Geometry check sheet. Reference: the model listing, model coordinates, mm. Face numbers are marked on the shaded views. Coordinates: 2 decimals unless noted, no trailing zeros. Write each loop counter-clockwise with the first axis right and the second up, starting at its lowest first coordinate (ties: lowest second). Pieces come first, ordered by that corner, then holes. Notation, with made-up numbers: (37.25, 70.5) - (64.25, 70.5) arc R21 ccw to (64.25, 94.5) - close; hole circle Ø9 at (-32, 71.5). An arc over 180 degrees is marked (long way). Answer as a JSON object with one key per item and string values. Group by question number.
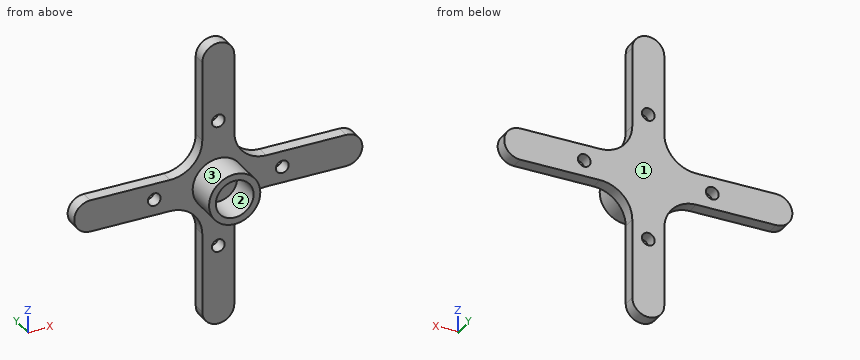
from build123d import *

# Parameters (mm, degrees)
SKETCH1_R           = 1
BOSS_EXTRUDE1_DEPTH = 2
SKETCH2_R           = 4
SKETCH2_R_2         = 2.95
BOSS_EXTRUDE2_DEPTH = 5


with BuildPart() as part:
    # Sketch1 → Boss-Extrude1 (new body)
    with BuildSketch(Plane(origin=(0, 0, 0), x_dir=(1, 0, 0), z_dir=(0, 1, 0))):
        with BuildLine():
            Line((2.5, 20), (2.5, 7.5))
            ThreePointArc((2.5, 7.5), (3.964466094, 3.964466094), (7.5, 2.5))
            Line((7.5, 2.5), (20, 2.5))
            ThreePointArc((20, 2.5), (22.5, 0), (20, -2.5))
            Line((20, -2.5), (7.5, -2.5))
            ThreePointArc((7.5, -2.5), (3.964466094, -3.964466094), (2.5, -7.5))
            Line((2.5, -7.5), (2.5, -20))
            ThreePointArc((2.5, -20), (0, -22.5), (-2.5, -20))
            Line((-2.5, -20), (-2.5, -7.5))
            ThreePointArc((-2.5, -7.5), (-3.964466094, -3.964466094), (-7.5, -2.5))
            Line((-7.5, -2.5), (-20, -2.5))
            ThreePointArc((-20, -2.5), (-22.5, 0), (-20, 2.5))
            Line((-20, 2.5), (-7.5, 2.5))
            ThreePointArc((-7.5, 2.5), (-3.964466094, 3.964466094), (-2.5, 7.5))
            Line((-2.5, 7.5), (-2.5, 20))
            ThreePointArc((-2.5, 20), (0, 22.5), (2.5, 20))
        make_face()
        with Locations(Location((10, 0, 0), (0, 0, 270))):
            Circle(SKETCH1_R, mode=Mode.SUBTRACT)
        with Locations(Location((-10, 0, 0), (0, 0, 270))):
            Circle(SKETCH1_R, mode=Mode.SUBTRACT)
        with Locations(Location((0, 10, 0), (0, 0, 270))):
            Circle(SKETCH1_R, mode=Mode.SUBTRACT)
        with Locations(Location((0, -10, 0), (0, 0, 270))):
            Circle(SKETCH1_R, mode=Mode.SUBTRACT)
    extrude(amount=BOSS_EXTRUDE1_DEPTH)

    # Sketch2 → Boss-Extrude2 (add)
    with BuildSketch(Plane.XZ):
        with Locations(Location((0, 0, 0), (0, 0, 90))):
            Circle(SKETCH2_R)
        with Locations(Location((0, 0, 0), (0, 0, 270))):
            Circle(SKETCH2_R_2, mode=Mode.SUBTRACT)
    extrude(amount=BOSS_EXTRUDE2_DEPTH)


solid = part.part
(1) Section check B-B (x = -10). Record the cut outline in (y, z), and give its area (3 significant figures).
(2) Draft check along Z on the marked faces 1, 2 and 3. Enter one of: +Z half, -Z half, draft (parallel to the pull), parting line (faces both ways), or undercut.
(3) Gauge pin test, flat ends, axial feed: pin 1 (2 mm diameter, centred on x = -14, y = 0.5, fed in from -Z); pin 2 (1.6 mm diameter, centred on x = 15, y = 1.5, fed in from +Z); pin 3 (1.6 mm diameter, centred on y = 1.5, z = 14.5, fed in from +X). Record the tip position at first contact, or that the pin passes through.
(4) Section check A-A (z = -10). Record the cut outline in (x, y), and give its area (3 significant figures).
(5) Section check D-D (x = 0). Record the cut outline in (y, z), and give its area (3 significant figures).
(6) Section check C-C (y = 0.75). Record the cut outline in (x, z), and give its area (3 significant figures).
(7) Material ranges on L1, parallel to X at y = 0.55, z = 0; L2, parallel to X at y = 1, z = 10; L3, parallel to X at y = -1.45, z = 0, recorded low to high. Write a range as [from, to].
Conclusion:
{
 "1": {"outline": "(0, -2.5) - (2, -2.5) - (2, -1) - (0, -1) - close; (0, 1) - (2, 1) - (2, 2.5) - (0, 2.5) - close", "area": "6.00 mm^2"},
 "2": {"face 1": "draft", "face 2": "undercut", "face 3": "parting line"},
 "3": {"pin 1": "stops at z = -2.5", "pin 2": "stops at z = 2.5", "pin 3": "stops at x = 2.5"},
 "4": {"outline": "(-2.5, 0) - (-1, 0) - (-1, 2) - (-2.5, 2) - close; (1, 0) - (2.5, 0) - (2.5, 2) - (1, 2) - close", "area": "6.00 mm^2"},
 "5": {"outline": "(-5, -4) - (0, -4) - (0, -9) - (2, -9) - (2, 9) - (0, 9) - (0, 4) - (-5, 4) - (-5, 2.95) - (0, 2.95) - (0, -2.95) - (-5, -2.95) - close; (0, -22.5) - (2, -22.5) - (2, -11) - (0, -11) - close; (0, 11) - (2, 11) - (2, 22.5) - (0, 22.5) - close", "area": "92.5 mm^2"},
 "6": {"outline": "(-20, -2.5) - (-7.5, -2.5) arc R5 cw to (-2.5, -7.5) - (-2.5, -20) arc R2.5 ccw to (2.5, -20) - (2.5, -7.5) arc R5 cw to (7.5, -2.5) - (20, -2.5) arc R2.5 ccw to (20, 2.5) - (7.5, 2.5) arc R5 cw to (2.5, 7.5) - (2.5, 20) arc R2.5 ccw to (-2.5, 20) - (-2.5, 7.5) arc R5 cw to (-7.5, 2.5) - (-20, 2.5) arc R2.5 ccw to start; hole circle Ø2 at (-10, 0); hole circle Ø2 at (0, -10); hole circle Ø2 at (0, 10); hole circle Ø2 at (10, 0)", "area": "423 mm^2"},
 "7": {"L1": "x = [-22.5, -11], [-9, 9], [11, 22.5]", "L2": "x = [-2.5, -1], [1, 2.5]", "L3": "x = [-4, -2.95], [2.95, 4]"}
}
